The listing builds one solid part. Answer for the finished solid, in the listing's coordinates (mm). Give positions to 0.01 mm unless a question says otherwise; leave off trailing zeros. Write each loop counter-clockwise with the first axis right and the second up, starting at its lowest first coordinate (ties: lowest second). Pieces come first, ordered by that corner, then holes. Notation, with made-up numbers: (2.5, 7.25) - (37.5, 7.25) arc R21 cw to (37.5, 41.25) - close; hole circle Ø6 at (27, -5.5). An arc over 180 degrees is marked (long way). One line per question, with ' | ' between items. Start each with the question number.
1. A cutting plane is placed at C-C (y = 0.2). State how many separate pieces and enclosed holes the cut face has, then the cut area to 3 significant figures.
2. A cutting plane is placed at D-D (x = 5.75). Determine the outline of the cut face in (y, z).
3. Find the intervals of material crossed by L1, parallel to X at y = 0.8, z = -11.25; L2, parallel to X at y = 0.9, z = 0; L3, parallel to X at y = 0.2, z = -4.75, in increasing order. Write a range as from..to.
4. A cutting plane is placed at A-A (z = -5). Determine the outline of the cut face in (x, y), then the cut area to 3 significant figures.
5. A cutting plane is placed at B-B (z = 4). Determine the outline of the cut face in (x, y).
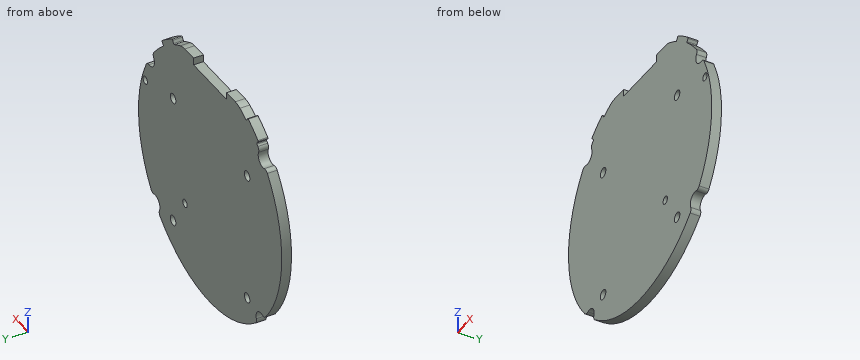
```python
from build123d import *

# Parameters (mm, degrees)
SKETCH1_R               = 13
BOSS_EXTRUDE1_DEPTH     = 1
CUT_EXTRUDE2_DEPTH      = 1
FILLET1_R               = 2
SKETCH4_R               = 0.5
CUT_EXTRUDE3_DEPTH      = 1
SKETCH6_R               = 0.85
CUT_EXTRUDE4_DEPTH      = 10
FILLET2_R               = 0.5
BOSS_EXTRUDE4_START     = -1
BOSS_EXTRUDE4_DEPTH     = 1
FILLET4_R               = 0.1
CUT_EXTRUDE6_DEPTH      = 19.411952786
CUT_EXTRUDE6_DEPTH_BACK = 19.411952786
SKETCH11_W              = 6
SKETCH11_H              = 1.5
SKETCH12_R              = 0.4
CUT_EXTRUDE7_DEPTH      = 1


with BuildPart() as part:
    # Sketch1 → Boss-Extrude1 (new body)
    with BuildSketch(Plane(origin=(0, 0, 0), x_dir=(1, 0, 0), z_dir=(0, 1, 0))):
        with Locations(Location((0, 0, 0), (0, 0, 270))):
            Circle(SKETCH1_R)
    extrude(amount=BOSS_EXTRUDE1_DEPTH)

    # Sketch3 → Cut-Extrude2 (cut)
    with BuildSketch(Plane(origin=(0, 0, 0), x_dir=(1, 0, 0), z_dir=(0, 1, 0))):
        with BuildLine():
            Line((-5, -12), (5, -12))
            ThreePointArc((5, -12), (0, -13), (-5, -12))
        make_face()
    extrude(amount=CUT_EXTRUDE2_DEPTH, mode=Mode.SUBTRACT)

    # Fillet1
    fillet1_edges = [part.edges().sort_by_distance(p)[0] for p in [
        (-5, 0.5, 12),
        (5, 0.5, 12),
    ]]
    fillet(fillet1_edges, radius=FILLET1_R)

    # Sketch4 → Cut-Extrude3 (cut)
    with BuildSketch(Plane.XZ):
        with Locations(Location((6.717514421, 5.186869411, 0), (0, 0, 270))):
            Circle(SKETCH4_R)
        with Locations(Location((-6.717514421, 5.186869411, 0), (0, 0, 270))):
            Circle(SKETCH4_R)
        with Locations(Location((-6.717514421, -8.248159431, 0), (0, 0, 270))):
            Circle(SKETCH4_R)
        with Locations(Location((6.717514421, -8.248159431, 0), (0, 0, 270))):
            Circle(SKETCH4_R)
    extrude(amount=-CUT_EXTRUDE3_DEPTH, mode=Mode.SUBTRACT)

    # Sketch6 → Cut-Extrude4 (cut)
    with BuildSketch(Plane.XZ):
        with Locations((9.958577761, -8.356238926)):
            Circle(SKETCH6_R)
        with Locations((-9.584605379, 8.782672699)):
            Circle(SKETCH6_R)
        with Locations((-9.192388155, -9.192388155)):
            Circle(SKETCH6_R)
        with Locations((10.964088796, 6.984894909)):
            Circle(SKETCH6_R)
    extrude(amount=-CUT_EXTRUDE4_DEPTH, mode=Mode.SUBTRACT)

    # Fillet2
    fillet2_edges = [part.edges().sort_by_distance(p)[0] for p in [
        (10.484191703, 0.5, 7.686463708),
        (11.397112787, 0.5, 6.25346465),
        (-10.138062294, 0.5, 8.137548337),
        (-8.990172858, 0.5, 9.390249836),
        (-8.57201926, 0.5, -9.773458232),
        (-9.773458232, 0.5, -8.57201926),
        (10.483367978, 0.5, -7.687587127),
        (9.39121315, 0.5, -8.989166567),
    ]]
    fillet(fillet2_edges, radius=FILLET2_R)

    # Sketch10 → Boss-Extrude4 (add)
    with BuildSketch(Plane(origin=(0, 1, 0), x_dir=(1, 0, 0), z_dir=(0, 1, 0)).offset(BOSS_EXTRUDE4_START)):
        with BuildLine():
            Line((-6.597998718, -11.201179086), (-6.8517679, -11.631993666))
            ThreePointArc((-6.8517679, -11.631993666), (-7.839489902, -10.990559498), (-8.767548652, -10.265480536))
            Line((-8.767548652, -10.265480536), (-8.442824628, -9.885277553))
            ThreePointArc((-8.442824628, -9.885277553), (-7.549138424, -10.583501739), (-6.597998718, -11.201179086))
        make_face()
        with BuildLine():
            Line((8.442824628, -9.885277553), (8.767548652, -10.265480536))
            ThreePointArc((8.767548652, -10.265480536), (7.839489902, -10.990559498), (6.8517679, -11.631993666))
            Line((6.8517679, -11.631993666), (6.597998718, -11.201179086))
            ThreePointArc((6.597998718, -11.201179086), (7.549138424, -10.583501739), (8.442824628, -9.885277553))
        make_face()
    extrude(amount=BOSS_EXTRUDE4_DEPTH)

    # Fillet4
    fillet4_edges = [part.edges().sort_by_distance(p)[0] for p in [
        (-8.442824628, 0.5, 9.885277553),
        (-6.597998718, 0.5, 11.201179086),
        (-6.8517679, 0.5, 11.631993666),
        (-8.767548652, 0.5, 10.265480536),
        (6.597998718, 0.5, 11.201179086),
        (8.442824628, 0.5, 9.885277553),
        (8.767548652, 0.5, 10.265480536),
        (6.8517679, 0.5, 11.631993666),
    ]]
    fillet(fillet4_edges, radius=FILLET4_R)

    # Sketch11 → Cut-Extrude6 (cut, two sides: drawn at the far end of the back side and taken through both)
    with BuildSketch(Plane(origin=(0, 0, 0), x_dir=(1, 0, 0), z_dir=(0, 1, 0)).offset(-CUT_EXTRUDE6_DEPTH_BACK)):
        with Locations((0, -12)):
            Rectangle(SKETCH11_W, SKETCH11_H)
    extrude(amount=CUT_EXTRUDE6_DEPTH + CUT_EXTRUDE6_DEPTH_BACK, mode=Mode.SUBTRACT)

    # Sketch12 → Cut-Extrude7 (cut)
    with BuildSketch(Plane(origin=(0, 1, 0), x_dir=(1, 0, 0), z_dir=(0, 1, 0))):
        with Locations(Location((4.571073678, 5, 0), (0, 0, 270))):
            Circle(SKETCH12_R)
        with Locations(Location((11.782754706, -4.000000001, 0), (0, 0, 270))):
            Circle(SKETCH12_R)
    extrude(amount=-CUT_EXTRUDE7_DEPTH, mode=Mode.SUBTRACT)


solid = part.part
```
Determined:
1) separate pieces: 1 | enclosed holes: 6 | area: 513 mm2
2) outline: (0, -11.66) - (1, -11.66) - (1, 11.66) - (0, 11.66) - close
3) L1: -6.51..6.51 | L2: -13..13 | L3: -12.1..4.26, 4.88..12.1
4) outline: (-12, 0) - (4.17, 0) - (4.17, 1) - (-12, 1) - close; (4.97, 0) - (12, 0) - (12, 1) - (4.97, 1) - close | area: 23.2 mm2
5) outline: (-12.37, 0) - (11.38, 0) - (11.38, 1) - (-12.37, 1) - close; (12.18, 0) - (12.37, 0) - (12.37, 1) - (12.18, 1) - close
